Autodesk Inventor part; units mm, degrees
ref_plane "YZ Plane" through (0, 0, 0) normal (1, 0, 0) x (0, 1, 0)
ref_plane "XZ Plane" through (0, 0, 0) normal (0, 1, 0) x (-1, 0, 0)
ref_plane "XY Plane" through (0, 0, 0) normal (0, 0, 1) x (1, 0, 0)
sketch "本体面" plane through (0, 0, 0) normal (0, 1, 0) x (-1, 0, 0)
  line L0 (20, 42) -> (-20, 42)
  line L1 (-20, 42) -> (-20, -42)
  line L2 (-20, -42) -> (20, -42)
  line L3 (20, -42) -> (20, 42)
  line L4 (20, 0) -> (-20, 0) construction
  line L5 (0, 42) -> (0, -42) construction
  point P0 (0, 0)
  point P1 (0, 0)
  dimension "d0" = 84
  dimension "d1" = 40
extrude "本体" add sketch "本体面" against normal blind 16
sketch "背羽形状" plane through (0, -16, 0) normal (0, -1, 0) x (1, 0, 0)
  line L0 (-20, -50) -> (-13, -50)
  line L1 (-8, -45) -> (-8, 45)
  line L2 (-13, 50) -> (-20, 50)
  line L3 (-20, 50) -> (-20, -50)
  line L4 (-20, 42) -> (-20, -42)
  arc A0 (-13, -50) -> (-8, -45) centre (-13, -45) ccw
  arc A1 (-8, 45) -> (-13, 50) centre (-13, 45) ccw
  point P0 (0, 0)
  point P1 (-8, 50)
  point P2 (-8, -50)
  point P3 (-20, 0)
  point P4 (-20, 50)
  point P5 (-20, -50)
  dimension "d94" = 100
  dimension "d95" = 12
  dimension "d128" = 5
extrude "背羽" add sketch "背羽形状" against normal blind 1.2
sketch "上羽形状" plane through (-20, 0, -42) normal (-1, 0, 0) x (0, 0, 1)
  line L0 (92, -16) -> (-8, -16)
  line L1 (-8, -16) -> (-8, -9)
  line L2 (-3, -4) -> (87, -4)
  line L3 (92, -9) -> (92, -16)
  line L4 (92, -16) -> (-8, -16)
  arc A0 (92, -9) -> (87, -4) centre (87, -9) ccw
  arc A1 (-3, -4) -> (-8, -9) centre (-3, -9) ccw
  point P0 (42, 0)
  point P1 (-8, -4)
  point P2 (92, -4)
  point P3 (42, -16)
  dimension "d122" = 100
  dimension "d123" = 12
  dimension "d124" = 5
  dimension "d125" = 5
extrude "上羽" add sketch "上羽形状" against normal blind 1.2
sketch "空洞上面" plane through (0, 0, 0) normal (0, 1, 0) x (1, 0, 0)
  line L0 (-19, -41) -> (19, -41)
  line L1 (19, -41) -> (19, 41)
  line L2 (19, 41) -> (-19, 41)
  line L3 (-19, 41) -> (-19, -41)
  line L4 (-19, 0) -> (19, 0) construction
  line L5 (0, -41) -> (0, 41) construction
  point P0 (0, 0)
  point P1 (0, 0)
  dimension "d4" = 82
  dimension "d5" = 38
extrude "空洞上" cut sketch "空洞上面" against normal blind 6
sketch "空洞下面" plane through (0, -6, 0) normal (0, 1, 0) x (1, 0, 0)
  line L0 (-13, -40) -> (13, -40)
  line L1 (18, -35) -> (18, 35)
  line L2 (13, 40) -> (-13, 40)
  line L3 (-18, 35) -> (-18, -35)
  line L4 (-18, 0) -> (18, 0) construction
  line L5 (0, -40) -> (0, 40) construction
  line L6 (-14, -35) -> (-18, -35)
  line L7 (-13, -36) -> (-13, -40)
  line L8 (14, -35) -> (18, -35)
  line L9 (13, -36) -> (13, -40)
  line L10 (-14, 35) -> (-18, 35)
  line L11 (-13, 36) -> (-13, 40)
  line L12 (14, 35) -> (18, 35)
  line L13 (13, 36) -> (13, 40)
  arc A0 (-13, -36) -> (-14, -35) centre (-14, -36) ccw
  arc A1 (14, -35) -> (13, -36) centre (14, -36) ccw
  arc A2 (-14, 35) -> (-13, 36) centre (-14, 36) ccw
  arc A3 (13, 36) -> (14, 35) centre (14, 36) ccw
  point P0 (0, 0)
  point P1 (0, 0)
  point P2 (-13, -35)
  point P3 (13, -35)
  point P4 (-13, 35)
  point P5 (13, 35)
  dimension "d10" = 36
  dimension "d11" = 80
  dimension "d12" = 5
  dimension "d13" = 5
  dimension "d14" = 5
  dimension "d15" = 5
  dimension "d16" = 5
  dimension "d17" = 5
  dimension "d18" = 5
  dimension "d19" = 5
  dimension "d20" = 1
extrude "空洞下" cut sketch "空洞下面" against normal blind 8
sketch "取付穴位置" plane through (0, -6, 0) normal (0, 1, 0) x (1, 0, 0)
  line L0 (0, 37.5) -> (0, -37.5) construction
  line L1 (-15.5, -37.5) -> (15.5, -37.5) construction
  line L2 (-15.5, 37.5) -> (15.5, 37.5) construction
  point P0 (0, 0)
  point P1 (0, 0)
  dimension "d26" = 75
  dimension "d27" = 31
  dimension "d28" = 31
hole "取付穴" at (-15.5, -6, 37.5) at (15.5, -6, 37.5) at (-15.5, -6, -37.5) at (15.5, -6, -37.5) direction (0, -1, 0) diameter 2.4 depth 20 tip angle 118
sketch "ケーブル穴右形状" plane through (20, 0, -42) normal (0, 0, -1) x (-1, 0, 0)
  line L0 (0, 0) -> (20, 0) construction
  line L1 (20, 0) -> (20, -8) construction
  line L2 (20, -4) -> (20, -12) construction
  line L3 (10, -4) -> (30, -4)
  line L4 (30, -4) -> (30, -12)
  line L5 (30, -12) -> (10, -12)
  line L6 (10, -12) -> (10, -4)
  line L7 (10, -4) -> (30, -12) construction
  line L8 (30, -4) -> (10, -12) construction
  point P0 (20, 0)
  point P1 (24, -8)
  dimension "d76" = 20
  dimension "d155" = 8
  dimension "d156" = 20
extrude "ケーブル穴右" cut sketch "ケーブル穴右形状" against normal blind 5
sketch "ケーブル穴左形状" plane through (-20, 0, 42) normal (0, 0, 1) x (1, 0, 0)
  line L0 (0, 0) -> (20, 0) construction
  line L1 (20, 0) -> (20, -8) construction
  line L2 (20, -4) -> (20, -12) construction
  line L3 (10, -4) -> (30, -4)
  line L4 (10, -12) -> (30, -12)
  line L5 (30, -12) -> (30, -4)
  line L6 (30, -4) -> (10, -4)
  line L7 (10, -4) -> (10, -12)
  line L8 (10, -12) -> (30, -4) construction
  line L9 (30, -12) -> (10, -4) construction
  point P0 (20, 0)
  dimension "d98" = 20
  dimension "d99" = 8
  dimension "d101" = 8
  dimension "d157" = 20
extrude "ケーブル穴左" cut sketch "ケーブル穴左形状" against normal blind 5
sketch "上穴位置" plane through (-20, 0, -42) normal (-1, 0, 0) x (0, 0, 1)
  line L0 (42, -16) -> (42, -10) construction
  line L1 (92, -16) -> (-8, -16) construction
  line L2 (86.45, -10) -> (-2.45, -10) construction
  point P0 (42, 0)
  dimension "d129" = 6
  dimension "d130" = 88.9
hole "上穴" at (-20, -10, 44.45) at (-20, -10, 0) at (-20, -10, -44.45) direction (1, 0, 0) diameter 2.5 depth 8 tip angle 118
sketch "背穴位置" plane through (0, -16, 0) normal (0, -1, 0) x (1, 0, 0)
  line L0 (-20, 0) -> (20, 0) construction
  line L1 (-20, 50) -> (-20, -50) construction
  line L2 (-14, -45) -> (-14, 45) construction
  line L3 (20, -42) -> (20, 42) construction
  point P0 (0, 0)
  point P1 (-14, 0)
  point P2 (0, 0)
  dimension "d139" = 90
  dimension "d147" = 6
hole "背穴" at (-14, -16, -45) at (-14, -16, 45) at (0, -16, 0) direction (0, 1, 0) diameter 2.5 depth 8 tip angle 118
properties part number "OLED_holder"
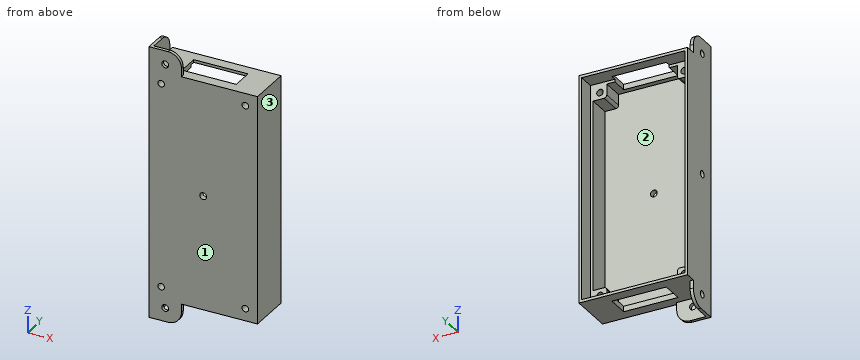
Check sheet for the modelled part. Datum: model origin and axes. Units: mm. Face numbers are marked on the shaded views. Give positions to 0.01 mm unless a question says otherwise; leave off trailing zeros. Loops run counter-clockwise (first coordinate to the right, second up) from the corner with the lowest first, then second, coordinate; pieces in that order, holes last. Notation, with made-up numbers: M 46,-21.5 L 72,-21.5 A23 cw 72,-5.5 Z; hole C 75,9 d2. An arc over 180 degrees is marked long. Use a Markdown table: item, result. Add a question column.
Q1. Sectioned sample at A-A, the plane z = 37.5. Record the cut outline in (x, y), then the cut area to 3 significant figures.
Q2. Sectioned sample at C-C, the plane x = 0. Record the cut outline in (y, z), then the cut area to 3 significant figures.
Q3. Sectioned sample at D-D, the plane y = -10. Give the number of separate pieces and of enclosed holes in the cut face, then the cut area to 3 significant figures.
Q4. Scan lines: line 1 along Z through (x, y) = (-15.5, -12.5); line 2 along X through (y, z) = (-12, -37.5); line 3 along X through (y, z) = (-1.75, 32). Record each from-to range of solid material in increasing order. Write a range as [from, to].
Q5. Sectioned sample at B-B, the plane x = 6.5. Record the cut outline in (y, z), then the cut area to 3 significant figures.
Q6. Go/stop test with flat-tipped pins: pin 1 (12 mm diameter, centred on x = 4.5, z = 26.5, fed in from +Y); pin 2 (5 mm diameter, centred on x = -14, y = -11.5, fed in from +Z); pin 3 (6.5 mm diameter, centred on x = -9, y = -3, fed in from -Z). Record where each tip stops, or that it passes through.
Q7. Mould release check, pull along Y, two halves, no side actions. Record for the marked faces 1, 2 and 3: pulls with the +Y half, pulls with the -Y half, needs draft (parallel to the pull), parting line crosses it, or undercut.
Verdict:
| question | item | result |
|---|---|---|
| 1 | outline | M -20,-16 L -16.7,-16 L -16.7,-6 L -19,-6 L -19,0 L -20,0 Z; M -14.3,-16 L 14.3,-16 L 14.3,-6 L 13,-6 L 13,-14 L -13,-14 L -13,-6 L -14.3,-6 Z; M 16.7,-16 L 20,-16 L 20,0 L 19,0 L 19,-6 L 16.7,-6 Z |
| 1 | area | 156 mm^2 |
| 2 | outline | M -16,-42 L -12,-42 L -12,-40 L -14,-40 L -14,-1.25 L -16,-1.25 Z; M -16,1.25 L -14,1.25 L -14,40 L -12,40 L -12,42 L -16,42 Z; M -4,-42 L 0,-42 L 0,-41 L -4,-41 Z; M -4,41 L 0,41 L 0,42 L -4,42 Z |
| 2 | area | 179 mm^2 |
| 3 | separate pieces | 5 |
| 3 | enclosed holes | 4 |
| 3 | area | 489 mm^2 |
| 4 | line 1 | [-42, -38.7], [-36.3, -35], [35, 36.3], [38.7, 42] |
| 4 | line 2 | [-20, -16.7], [-14.3, -13], [13, 14.3], [16.7, 20] |
| 4 | line 3 | [-20, -19], [19, 20] |
| 5 | outline | M -16,-42 L -12,-42 L -12,-40 L -14,-40 L -14,40 L -12,40 L -12,42 L -16,42 Z; M -4,-42 L 0,-42 L 0,-41 L -4,-41 Z; M -4,41 L 0,41 L 0,42 L -4,42 Z |
| 5 | area | 184 mm^2 |
| 6 | pin 1 | y = -14 |
| 6 | pin 2 | z = 42 |
| 6 | pin 3 | z = -42 |
| 7 | face 1 | pulls with the -Y half |
| 7 | face 2 | pulls with the +Y half |
| 7 | face 3 | needs draft |
